The model under review builds one solid part; all positions refer to its coordinate system, in mm. A direction names the side the tool comes from. Round coordinates to 2 decimals unless told otherwise and drop trailing zeros. Answer as a JSON object with one key per item and string values. Group by question number.
Item 1: Insertion check: P1, Ø5, axis at x = 503, z = -85.5, coming from the +Y side; P2, Ø4.5, axis at x = 503, y = -1260.5, coming from the -Z side; P3, Ø1.5, axis at x = 501.5, y = -1203.5, coming from the -Z side. Each pin has a flat end and moves straight along its axis. Give the tip position at first contact, or say it passes through.
Item 2: To check wall thickness, follow line 1 (Y direction, x = 503.75, z = -101.5); line 2 (Z direction, x = 502.75, y = -1190); line 3 (Z direction, x = 505.75, y = -1188.5). State the ranges of each line that lie inside material, in increasing order.
Item 3: The part is to be moulded in two halves that separate along Y. For faces 1 (the face through (496, -1215, -128)), 2 (the face through (500.93, -1180.83, -139.2)), 3 (the face through (501, -1264, -101)), 4 (the face through (501, -1230.49, -86)), say which applies: +Y half, -Y half, draft (parallel to the pull), parting line (faces both ways), or undercut.
Item 4: Tool access review of faces 5 (the face through (500.93, -1239.645, -88.658)), 6 (the face through (500.93, -1269.7, -145.22)), 7 (the face through (500.93, -1244.94, -165.31)), 8 (the face through (500.93, -1240.673, -166.768)): name each direction out of +Z, -Z, +X, -X, +Y, -Y from which nothing blocks a thin tool from reaching the whole face with its end or side.
```python
from build123d import *

# Parameters (mm, degrees)
SKETCH002_R  = 7.5
PAD001_DEPTH = 10


with BuildPart() as part:
    # Sketch002 → Pad001 (new body)
    with BuildSketch(Plane.YZ):
        with BuildLine():
            ThreePointArc((-7.372881, -40.094264), (-3.126041, -39.586192), (1.04227, -38.627568))
            Line((1.04227, -38.627568), (0.551182, -41.772804))
            ThreePointArc((0.551182, -41.772804), (2.72771, -45.044909), (6.248691, -46.790371))
            ThreePointArc((6.248691, -46.790371), (7.994153, -43.26939), (7.745277, -39.3474))
            Line((5.322974, -37.131356), (7.745277, -39.3474))
            ThreePointArc((5.322974, -37.131356), (8.537274, -35.628587), (11.605754, -33.846883))
            Line((11.605754, -33.846883), (12.333348, -38.63991))
            ThreePointArc((12.333348, -38.63991), (15.097939, -41.134767), (18.739574, -41.913081))
            ThreePointArc((18.739574, -41.913081), (19.517888, -38.271446), (18.37111, -34.728541))
            Line((14.654104, -31.683604), (18.37111, -34.728541))
            ThreePointArc((14.654104, -31.683604), (17.378229, -29.347876), (19.882066, -26.777412))
            Line((19.882066, -26.777412), (21.219608, -30.122295))
            ThreePointArc((21.219608, -30.122295), (24.552318, -31.581454), (28.168109, -31.178768))
            ThreePointArc((28.168109, -31.178768), (27.765423, -27.562977), (25.608791, -24.632953))
            Line((22.518982, -23.480322), (25.608791, -24.632953))
            ThreePointArc((22.518982, -23.480322), (23.893543, -21.431633), (25.139192, -19.302101))
            Line((25.139192, -19.302101), (27.359533, -21.66958))
            ThreePointArc((27.359533, -21.66958), (31.317426, -23.081877), (35.451211, -22.326017))
            ThreePointArc((35.451211, -22.326017), (34.69535, -18.192232), (31.973863, -14.9902))
            Line((27.63708, -13.740754), (31.973863, -14.9902))
            ThreePointArc((27.63708, -13.740754), (28.311222, -11.699588), (28.874738, -9.625154))
            Line((28.874738, -9.625154), (31.548764, -11.314179))
            ThreePointArc((31.548764, -11.314179), (35.22362, -11.182883), (38.340491, -9.231748))
            ThreePointArc((38.340491, -9.231748), (36.389357, -6.114877), (33.141189, -4.391155))
            Line((29.744589, -4.744157), (33.141189, -4.391155))
            ThreePointArc((29.744589, -4.744157), (29.958098, -2.133322), (30.00026, 0.485889))
            Line((30.00026, 0.485889), (33.921496, -0.257635))
            ThreePointArc((33.921496, -0.257635), (37.68409, 0.725166), (40.451192, 3.457594))
            ThreePointArc((40.451192, 3.457594), (37.718763, 6.224696), (33.968861, 7.254862))
            Line((29.545098, 5.873223), (33.968861, 7.254862))
            ThreePointArc((29.545098, 5.873223), (29.208197, 7.767875), (28.780562, 9.644132))
            Line((28.780562, 9.644132), (33.177289, 10.00993))
            ThreePointArc((33.177289, 10.00993), (35.728214, 11.395702), (37.244494, 13.871278))
            ThreePointArc((37.244494, 13.871278), (34.768918, 15.387558), (31.866866, 15.462907))
            Line((27.436049, 13.925673), (31.866866, 15.462907))
            ThreePointArc((27.436049, 13.925673), (26.375433, 16.470589), (25.142027, 18.936397))
            Line((25.142027, 18.936397), (29.967849, 21.069522))
            ThreePointArc((29.967849, 21.069522), (31.970773, 23.393509), (32.543362, 26.407602))
            ThreePointArc((32.543362, 26.407602), (29.529269, 26.980191), (26.632693, 25.969022))
            Line((22.726486, 22.827517), (26.632693, 25.969022))
            ThreePointArc((22.726486, 22.827517), (20.942152, 25.176066), (18.98961, 27.386747))
            Line((18.98961, 27.386747), (22.859671, 29.824034))
            ThreePointArc((22.859671, 29.824034), (24.506903, 32.07831), (24.80631, 34.854187))
            ThreePointArc((24.80631, 34.854187), (22.030434, 35.153594), (19.476751, 34.02495))
            Line((16.440698, 29.839688), (19.476751, 34.02495))
            ThreePointArc((16.440698, 29.839688), (14.740616, 31.25523), (12.964876, 32.574618))
            Line((12.964876, 32.574618), (16.319999, 35.447081))
            ThreePointArc((16.319999, 35.447081), (16.941471, 38.969468), (15.718489, 42.330681))
            ThreePointArc((15.718489, 42.330681), (12.357276, 41.107698), (10.057871, 38.367958))
            Line((9.433448, 34.784975), (10.057871, 38.367958))
            ThreePointArc((9.433448, 34.784975), (7.223624, 35.924417), (4.947279, 36.924367))
            Line((4.947279, 36.924367), (7.1719, 40.70615))
            ThreePointArc((7.1719, 40.70615), (7.147067, 44.138089), (5.409592, 47.097818))
            ThreePointArc((5.409592, 47.097818), (2.449862, 45.360343), (0.755399, 42.37578))
            Line((0.780338, 38.341298), (0.755399, 42.37578))
            ThreePointArc((0.780338, 38.341298), (-1.831547, 38.978037), (-4.480302, 39.437893))
            Line((-4.480302, 39.437893), (-2.979924, 44.013792))
            ThreePointArc((-2.979924, 44.013792), (-4.253731, 47.105339), (-6.902654, 49.145794))
            ThreePointArc((-6.902654, 49.145794), (-8.943109, 46.496871), (-9.385733, 43.182609))
            Line((-8.16746, 39.778019), (-9.385733, 43.182609))
            ThreePointArc((-8.16746, 39.778019), (-11.333059, 39.797339), (-14.490272, 39.566265))
            Line((-14.490272, 39.566265), (-14.490272, 43.98748))
            ThreePointArc((-14.490272, 43.98748), (-15.999307, 47.081093), (-18.852977, 49.005722))
            ThreePointArc((-18.852977, 49.005722), (-20.777606, 46.152053), (-21.01755, 42.718388))
            Line((-18.483952, 38.908421), (-21.01755, 42.718388))
            ThreePointArc((-18.483952, 38.908421), (-20.883273, 38.309075), (-23.240971, 37.562604))
            Line((-23.240971, 37.562604), (-24.06091, 41.171638))
            ThreePointArc((-24.06091, 41.171638), (-26.267629, 43.82088), (-29.503325, 45.011832))
            ThreePointArc((-29.503325, 45.011832), (-30.694276, 41.776136), (-30.107822, 38.378465))
            Line((-26.761898, 36.135645), (-30.107822, 38.378465))
            ThreePointArc((-26.761898, 36.135645), (-29.419041, 34.786526), (-31.968369, 33.24333))
            Line((-31.968369, 33.24333), (-33.870535, 37.498149))
            ThreePointArc((-33.870535, 37.498149), (-37.164485, 39.463014), (-40.999563, 39.517661))
            ThreePointArc((-40.999563, 39.517661), (-41.05421, 35.682584), (-39.183997, 32.333986))
            Line((-35.835479, 30.35216), (-39.183997, 32.333986))
            ThreePointArc((-35.835479, 30.35216), (-37.957964, 28.420932), (-39.93653, 26.342505))
            Line((-39.93653, 26.342505), (-41.575001, 29.566843))
            ThreePointArc((-41.575001, 29.566843), (-44.88038, 30.944013), (-48.431509, 30.483987))
            ThreePointArc((-48.431509, 30.483987), (-47.971483, 26.932859), (-45.797525, 24.087505))
            Line((-41.791617, 24.087505), (-45.797525, 24.087505))
            ThreePointArc((-41.791617, 24.087505), (-44.160781, 20.619854), (-46.153311, 16.922914))
            Line((-46.153311, 16.922914), (-50.742028, 19.632063))
            ThreePointArc((-50.742028, 19.632063), (-54.205982, 19.16463), (-56.972138, 17.027844))
            ThreePointArc((-56.972138, 17.027844), (-54.835352, 14.261689), (-51.601763, 12.934521))
            Line((-47.669302, 13.257985), (-51.601763, 12.934521))
            ThreePointArc((-47.669302, 13.257985), (-48.596186, 10.30241), (-49.291589, 7.283975))
            Line((-49.291589, 7.283975), (-52.532451, 8.985395))
            ThreePointArc((-52.532451, 8.985395), (-55.852169, 8.811227), (-58.640045, 7.000533))
            ThreePointArc((-58.640045, 7.000533), (-56.829351, 4.212658), (-53.867307, 2.703633))
            Line((-49.801546, 3.740797), (-53.867307, 2.703633))
            ThreePointArc((-49.801546, 3.740797), (-49.982641, 0.781001), (-49.943969, -2.184078))
            Line((-49.943969, -2.184078), (-54.793138, -1.899745))
            ThreePointArc((-54.793138, -1.899745), (-58.035986, -3.927121), (-59.830686, -7.304304))
            ThreePointArc((-59.830686, -7.304304), (-56.453504, -9.099004), (-52.631427, -8.964669))
            Line((-49.409647, -6.993613), (-52.631427, -8.964669))
            ThreePointArc((-49.409647, -6.993613), (-48.670532, -10.385186), (-47.640158, -13.69991))
            Line((-47.640158, -13.69991), (-50.982572, -14.298306))
            ThreePointArc((-50.982572, -14.298306), (-53.725014, -17.270261), (-54.614061, -21.21527))
            ThreePointArc((-54.614061, -21.21527), (-50.669052, -22.104317), (-46.808051, -20.90175))
            Line((-45.349568, -18.888466), (-46.808051, -20.90175))
            ThreePointArc((-45.349568, -18.888466), (-43.812217, -21.542392), (-42.076041, -24.070726))
            Line((-42.076041, -24.070726), (-45.563033, -26.35824))
            ThreePointArc((-45.563033, -26.35824), (-46.88137, -30.023623), (-46.405266, -33.889676))
            ThreePointArc((-46.405266, -33.889676), (-42.308675, -33.202292), (-39.189808, -30.458714))
            Line((-38.622542, -28.116203), (-39.189808, -30.458714))
            ThreePointArc((-38.622542, -28.116203), (-35.930016, -30.632391), (-33.017345, -32.8901))
            Line((-33.017345, -32.8901), (-35.637207, -35.045193))
            ThreePointArc((-35.637207, -35.045193), (-36.797466, -38.717464), (-35.966145, -42.477874))
            ThreePointArc((-35.966145, -42.477874), (-32.205735, -41.646553), (-29.364786, -39.046402))
            Line((-28.526262, -35.628271), (-29.364786, -39.046402))
            ThreePointArc((-28.526262, -35.628271), (-26.329852, -36.692522), (-24.072624, -37.620837))
            Line((-24.072624, -37.620837), (-25.290637, -39.948337))
            ThreePointArc((-25.290637, -39.948337), (-25.224166, -44.200892), (-23.040323, -47.850478))
            ThreePointArc((-23.040323, -47.850478), (-19.390737, -45.666635), (-17.322024, -41.950579))
            Line((-18.195367, -39.33048), (-17.322024, -41.950579))
            ThreePointArc((-18.195367, -39.33048), (-15.388372, -39.814864), (-12.554022, -40.098254))
            Line((-12.554022, -40.098254), (-14.133284, -42.536876))
            ThreePointArc((-14.133284, -42.536876), (-13.138594, -46.750559), (-10.168772, -49.900906))
            ThreePointArc((-10.168772, -49.900906), (-6.910841, -46.753818), (-5.771565, -42.36972))
            Line((-7.372881, -40.094264), (-5.771565, -42.36972))
        make_face()
        with Locations((-9.994192, -0.180247)):
            Circle(SKETCH002_R, mode=Mode.SUBTRACT)
    extrude(amount=PAD001_DEPTH)


with BuildPart() as part_1:
    # Body001 placement: moved
    add(part.part.moved(Location((496, -1216, -128))))


solid = part_1.part
```
Geometry results:
{
 "1": {"P1": "stops at y = -1199.23", "P2": "stops at z = -161.94", "P3": "stops at z = -167.78"},
 "2": {"line 1": "y = -1263.78 to -1256.02, -1255.8 to -1196.19, -1188.41 to -1183.66", "line 2": "z = -159.65 to -152.97, -148.22 to -110.73, -108.68 to -102.54", "line 3": "z = -159.4 to -154.97, -149.76 to -114.05, -108.02 to -101.54"},
 "3": {"face 1": "draft", "face 2": "undercut", "face 3": "-Y half", "face 4": "undercut"},
 "4": {"face 5": "+Z, +X, -X", "face 6": "+X, -X, -Y", "face 7": "-Z, +X, -X", "face 8": "+X, -X"}
}
